Source: CAD feature listing. Evaluate the final solid. Frame: model axes, mm. A direction names the side the tool comes from. Round coordinates to 2 decimals unless told otherwise and drop trailing zeros. Write each loop counter-clockwise with the first axis right and the second up, starting at its lowest first coordinate (ties: lowest second). Pieces come first, ordered by that corner, then holes.
```python
from build123d import *

# Parameters (mm, degrees)
SKETCH1_R           = 3.25
SKETCH1_R_2         = 1.75
BOSS_EXTRUDE1_DEPTH = 3
SKETCH5_W           = 10
SKETCH5_H           = 9
CUT_EXTRUDE1_DEPTH  = 1.75


with BuildPart() as part:
    # Sketch1 → Boss-Extrude1 (new, symmetric)
    with BuildSketch(Plane.XY):
        with BuildLine():
            Line((-10, 4.5), (10, 4.5))
            ThreePointArc((10, 4.5), (14.5, 0), (10, -4.5))
            Line((10, -4.5), (-10, -4.5))
            ThreePointArc((-10, -4.5), (-14.5, 0), (-10, 4.5))
        make_face()
        with Locations((-10, 0)):
            Circle(SKETCH1_R, mode=Mode.SUBTRACT)
        with Locations((10, 0)):
            Circle(SKETCH1_R_2, mode=Mode.SUBTRACT)
    extrude(amount=BOSS_EXTRUDE1_DEPTH, both=True)

    # Sketch5 → Cut-Extrude1 (cut, symmetric)
    with BuildSketch(Plane.XY):
        with Locations((9.5, 0)):
            Rectangle(SKETCH5_W, SKETCH5_H)
    extrude(amount=CUT_EXTRUDE1_DEPTH, both=True, mode=Mode.SUBTRACT)


solid = part.part
```
Q1. Section query D-D, the plane z = 2.25. Output: boundary loops of the cut face in (x, y), and give its area (3 significant figures).
Q2. Section query B-B, the plane y = -0.75. Output: boundary loops of the cut face in (x, z), and give its area (3 significant figures).
Q3. Mould query, pull axis Y, two halves, no side actions, for faces 1 (the face through (-14.5, -0.1, 0)), 2 (the face through (11.669, 0.526, 2.366)), 3 (the face through (8, -1, 1.75)). Classes: pulls with the +Y half, pulls with the -Y half, needs draft (parallel to the pull), parting line crosses it, or undercut.
Q4. Section query A-A, the plane x = 6. Output: boundary loops of the cut face in (y, z).
Q5. Pin query (flat end, axial travel): P1, Ø1, axis at y = -3, z = 2, coming from the -X side; P2, Ø3, axis at y = -3, z = 1.5, coming from the +X side. Return the tip coordinate at first contact, or that it passes through.
Q6. Line query: line 1 (Y direction, x = 10, z = 2.65); line 2 (X direction, y = -0.25, z = 2.4); line 3 (X direction, y = -1, z = -2). Output: solid intervals per line, ascending.
Q7. Set-up query: faces 4 (the face through (4.5, 0, 0)), 5 (the face through (11.669, 0.526, -2.384)). Return all of +Z, -Z, +X, -X, +Y, -Y with unobstructed straight access to the full face (end or side cutting, diameter ignored); none if empty.
Q8. Section query C-C, the plane y = -2.5. Output: boundary loops of the cut face in (x, z), and give its area (3 significant figures).
Filled in:
1. outline: (-10, -4.5) - (10, -4.5) arc R4.5 ccw to (10, 4.5) - (-10, 4.5) arc R4.5 ccw to start; hole circle Ø6.5 at (-10, 0); hole circle Ø3.5 at (10, 0)
1. area: 201 mm2
2. outline: (-14.44, -3) - (-13.16, -3) - (-13.16, 3) - (-14.44, 3) - close; (-6.84, -3) - (8.42, -3) - (8.42, -1.75) - (4.5, -1.75) - (4.5, 1.75) - (8.42, 1.75) - (8.42, 3) - (-6.84, 3) - close; (11.58, -3) - (14.44, -3) - (14.44, -1.75) - (11.58, -1.75) - close; (11.58, 1.75) - (14.44, 1.75) - (14.44, 3) - (11.58, 3) - close
2. area: 92.6 mm2
3. face 1: parting line crosses it
3. face 2: undercut
3. face 3: needs draft
4. outline: (-4.5, -3) - (4.5, -3) - (4.5, -1.75) - (-4.5, -1.75) - close; (-4.5, 1.75) - (4.5, 1.75) - (4.5, 3) - (-4.5, 3) - close
5. P1: stops at x = -13.74
5. P2: stops at x = 14.24
6. line 1: y = -4.5 to -1.75, 1.75 to 4.5
6. line 2: x = -14.49 to -13.24, -6.76 to 8.27, 11.73 to 14.49
6. line 3: x = -14.39 to -13.09, -6.91 to 8.56, 11.44 to 14.39
7. face 4: +X, +Y, -Y
7. face 5: +Z, -Z
8. outline: (-13.74, -3) - (-12.08, -3) - (-12.08, 3) - (-13.74, 3) - close; (-7.92, -3) - (13.74, -3) - (13.74, -1.75) - (4.5, -1.75) - (4.5, 1.75) - (13.74, 1.75) - (13.74, 3) - (-7.92, 3) - close
8. area: 108 mm2
